from build123d import *

# Parameters (mm, degrees)
AUFSATZ_LINEAR_AUSTRAGEN1_DEPTH  = 20
SCHNITT_LINEAR_AUSTRAGEN2_REACH  = 2.5
SKIZZE8_W                        = 11
SKIZZE8_H                        = 5
AUFSATZ_LINEAR_AUSTRAGEN3_DEPTH  = 8.34
SCHNITT_LINEAR_AUSTRAGEN3_REACH  = 19.821
SKIZZE12_W                       = 1.5
SKIZZE12_H                       = 2
AUFSATZ_LINEAR_AUSTRAGEN4_DEPTH  = 3.98
AUFSATZ_LINEAR_AUSTRAGEN5_DEPTH  = 2.67
AUFSATZ_LINEAR_AUSTRAGEN6_DEPTH  = 2.67
SCHNITT_LINEAR_AUSTRAGEN4_REACH  = 23.901
SKIZZE17_W                       = 3
SKIZZE17_H                       = 16.288675134
AUFSATZ_LINEAR_AUSTRAGEN15_DEPTH = 6.65
SCHNITT_LINEAR_AUSTRAGEN5_REACH  = 14.32


with BuildPart() as part:
    # Skizze1 → Aufsatz-Linear austragen1 (new body)
    with BuildSketch(Plane(origin=(0, 0, 0), x_dir=(1, 0, 0), z_dir=(0, 1, 0))):
        Polygon((5.5, -4.17), (-5.5, -4.17), (-5.5, -1.5), (-7.5, -1.5), (-7.5, 1.5), (-5.5, 1.5), (-5.5, 4.17), (5.5, 4.17), (5.5, 1.5), (7.5, 1.5), (7.5, -1.5), (5.5, -1.5), align=None)
        Polygon((-5, 1), (-5, 3.67), (5, 3.67), (5, 1), (7, 1), (7, -1), (5, -1), (5, -3.67), (-5, -3.67), (-5, -1), (-7, -1), (-7, 1), align=None, mode=Mode.SUBTRACT)
    extrude(amount=AUFSATZ_LINEAR_AUSTRAGEN1_DEPTH)

    # Skizze8 → Schnitt-Linear austragen2 (cut, up to next)
    with BuildSketch(Plane(origin=(0, 0, 3.67), x_dir=(-1, 0, 0), z_dir=(0, 0, -1)), mode=Mode.PRIVATE) as schnitt_linear_austragen2_sk1:
        with Locations((0, 2.5)):
            Rectangle(SKIZZE8_W, SKIZZE8_H)
    schnitt_linear_austragen2_tool1 = extrude(schnitt_linear_austragen2_sk1.sketch, amount=-SCHNITT_LINEAR_AUSTRAGEN2_REACH, mode=Mode.PRIVATE) & part.part
    add(schnitt_linear_austragen2_tool1.solids().sort_by_distance((0, 2.5, 3.67))[0], mode=Mode.SUBTRACT)

    # Skizze10 → Aufsatz-Linear austragen3 (add)
    with BuildSketch(Plane(origin=(0, 0, -4.17), x_dir=(-1, 0, 0), z_dir=(0, 0, -1))):
        Polygon((5.5, 20), (7.211324865, 20), (17.211324865, 37.320508076), (17.644337567, 37.070508076), (7.5, 19.5), (5.5, 19.5), align=None)
    extrude(amount=-AUFSATZ_LINEAR_AUSTRAGEN3_DEPTH)

    # Skizze12 → Schnitt-Linear austragen3 (cut, up to next)
    with BuildSketch(Plane.XZ.offset(-19.5), mode=Mode.PRIVATE) as schnitt_linear_austragen3_sk1:
        with Locations((-6.25, 0)):
            Rectangle(SKIZZE12_W, SKIZZE12_H)
    schnitt_linear_austragen3_tool1 = extrude(schnitt_linear_austragen3_sk1.sketch, amount=-SCHNITT_LINEAR_AUSTRAGEN3_REACH, mode=Mode.PRIVATE) & part.part
    add(schnitt_linear_austragen3_tool1.solids().sort_by_distance((-6.25, 19.5, 0))[0], mode=Mode.SUBTRACT)

    # Skizze13 → Aufsatz-Linear austragen4 (add)
    with BuildSketch(Plane(origin=(0, 0, -4.17), x_dir=(-1, 0, 0), z_dir=(0, 0, -1))):
        Polygon((17.211324865, 37.320508076), (9.561324865, 24.070319398), (9.994337567, 23.820319398), (17.644337567, 37.070508076), align=None)
    aufsatz_linear_austragen4 = extrude(amount=AUFSATZ_LINEAR_AUSTRAGEN4_DEPTH)

    # Skizze15 → Aufsatz-Linear austragen5 (add)
    with BuildSketch(Plane(origin=(0, 0, -1.5), x_dir=(-1, 0, 0), z_dir=(0, 0, -1))):
        Polygon((5.5, 8), (5.5, 19.5), (7.5, 19.5), (17.644337567, 37.070508076), (7.5, 8), align=None)
    extrude(amount=AUFSATZ_LINEAR_AUSTRAGEN5_DEPTH)

    # Spiegeln1: Aufsatz-Linear austragen4 across plane
    add(aufsatz_linear_austragen4.mirror(Plane.XY))

    # Skizze16 → Aufsatz-Linear austragen6 (add)
    with BuildSketch(Plane.XY.offset(1.5)):
        Polygon((-17.644337567, 37.070508076), (-7.5, 8), (-5.5, 8), (-5.5, 19.5), (-7.5, 19.5), align=None)
    extrude(amount=AUFSATZ_LINEAR_AUSTRAGEN6_DEPTH)

    # Skizze17 → Schnitt-Linear austragen4 (cut, up to next)
    with BuildSketch(Plane(origin=(2.818747687, 1.627404736, 0), x_dir=(0, 0, 1), z_dir=(-0.866025404, -0.5, 0)), mode=Mode.PRIVATE) as schnitt_linear_austragen4_sk1:
        with Locations((0, 28.781832941)):
            Rectangle(SKIZZE17_W, SKIZZE17_H)
    schnitt_linear_austragen4_tool1 = extrude(schnitt_linear_austragen4_sk1.sketch, amount=-SCHNITT_LINEAR_AUSTRAGEN4_REACH, mode=Mode.PRIVATE) & part.part
    add(schnitt_linear_austragen4_tool1.solids().sort_by_distance((-11.572169, 26.553203, 0))[0], mode=Mode.SUBTRACT)

    # Skizze22 → Aufsatz-Linear austragen15 (add)
    with BuildSketch(Plane.XY.offset(-1.5)):
        Polygon((-17.611390326, 36.976091556), (-12.603409607, 22.624780496), (-13.075492208, 22.460044288), (-18.083472926, 36.811355348), align=None)
    aufsatz_linear_austragen15 = extrude(amount=-AUFSATZ_LINEAR_AUSTRAGEN15_DEPTH)

    # Spiegeln2: Aufsatz-Linear austragen15 across plane
    add(aufsatz_linear_austragen15.mirror(Plane.XY))

    # Skizze23 → Schnitt-Linear austragen5 (cut, up to next)
    with BuildSketch(Plane.XY.offset(4.17), mode=Mode.PRIVATE) as schnitt_linear_austragen5_sk1:
        Polygon((-7.211324865, 20), (-9.561324865, 20), (-9.561324865, 24.070319398), align=None)
    schnitt_linear_austragen5_tool1 = extrude(schnitt_linear_austragen5_sk1.sketch, amount=-SCHNITT_LINEAR_AUSTRAGEN5_REACH, mode=Mode.PRIVATE) & part.part
    add(schnitt_linear_austragen5_tool1.solids().sort_by_distance((-8.777992, 21.356773, 4.17))[0], mode=Mode.SUBTRACT)


solid = part.part
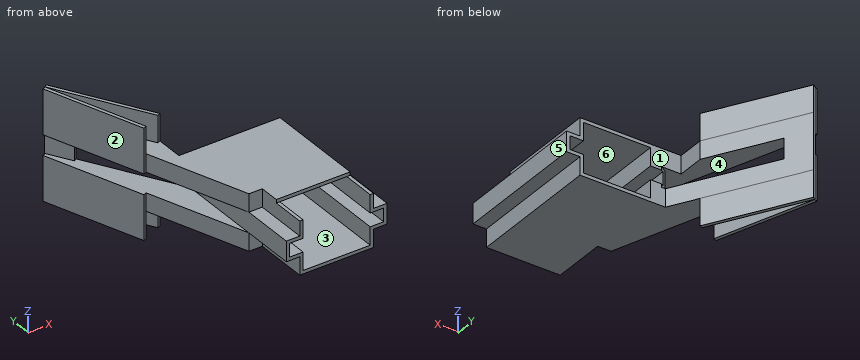
Verification items for the finished model (mm, model axes). Face numbers are marked on the shaded views. A direction names the side the tool comes from. Coordinates: 2 decimals unless noted, no trailing zeros. Order: outer loops, then holes, each group sorted by start corner. A loop starts at its lowest first (then second) coordinate and runs counter-clockwise, first axis right, second up. Notation, with made-up numbers: M 2.25,41 L 50.25,41 A21 cw 50.25,64 Z; hole C 72.5,66 d1. An arc over 180 degrees is marked long. One line per item, written item: value. Start each with the question number.
Item 1: Sectioned sample at B-B (z = -3). Enter the section's corners in (x, y).
Item 2: Sectioned sample at C-C (x = -3). Enter the section's corners in (y, z), then the cut area to 3 significant figures.
Item 3: Gauge pin test, flat ends, axial feed: pin 1 (0.8 mm diameter, centred on y = 10, z = 3, fed in from -X); pin 2 (0.8 mm diameter, centred on y = 22, z = 3, fed in from +X); pin 3 (1 mm diameter, centred on y = 29, z = 0, fed in from +X); pin 4 (8 mm diameter, centred on y = 32, z = -5.5, fed in from -X). Record the tip position at first contact, or that the pin passes through.
Item 4: Scan lines: probe 1 along X at (y, z) = (18, 0.5); probe 2 along X at (y, z) = (3.5, -1.25); probe 3 along Z at (x, y) = (-3.5, 12). Record each from-to range of solid material in increasing order.
Item 5: Mould release check, pull along X, two halves, no side actions. Record for the marked faces 3, 4, 5 and 6: released by +X, released by -X, zero draft, split by the parting line, or undercut.
Item 6: Access from +Z, -Z, +X, -X, +Y, -Y to the whole of each face (thin tool, end or side, straight path). Record for the marked faces 1 and 2.
Item 7: Sectioned sample at A-A (y = 7). Enter the section's corners in (x, z).
Item 8: Sectioned sample at D-D (y = 28.5). Enter the section's corners in (x, z), then the cut area to 3 significant figures.
Conclusion:
1. outline: M -18.08,36.81 L -13.08,22.46 L -12.6,22.62 L -7.5,8 L -5.5,8 L -5.5,0 L -5,0 L -5,20 L -7.21,20 L -17.21,37.32 L -17.64,37.07 L -17.61,36.98 Z; M 5,0 L 5.5,0 L 5.5,20 L 5,20 Z
2. outline: M 0,-4.17 L 20,-4.17 L 20,-3.67 L 0,-3.67 Z; M 5,3.67 L 20,3.67 L 20,4.17 L 5,4.17 Z
2. area: 17.5 mm^2
3. pin 1: stops at x = -8.34
3. pin 2: stops at x = -9.56
3. pin 3: passes through
3. pin 4: stops at x = -17.8
4. probe 1: x = -7.5 to -7, 7 to 7.5
4. probe 2: x = -7.5 to -5, 5 to 7.5
4. probe 3: z = -4.17 to -3.67, 3.67 to 4.17
5. face 3: undercut
5. face 4: zero draft
5. face 5: released by +X
5. face 6: undercut
6. face 1: +Z, +X, +Y
6. face 2: +Z, -Z, -X, -Y
7. outline: M -7.5,-1.5 L -5.5,-1.5 L -5.5,-4.17 L 5.5,-4.17 L 5.5,-1.5 L 7.5,-1.5 L 7.5,1.5 L 5.5,1.5 L 5.5,4.17 L -5.5,4.17 L -5.5,1.5 L -7.5,1.5 Z; hole M -7,-1 L -5,-1 L -5,-3.67 L 5,-3.67 L 5,-1 L 7,-1 L 7,1 L 5,1 L 5,3.67 L -5,3.67 L -5,1 L -7,1 Z
8. outline: M -15.18,-8.15 L -14.65,-8.15 L -14.65,-4.17 L -12.7,-4.17 L -12.7,-8.15 L -12.12,-8.15 L -12.12,-1.5 L -15.18,-1.5 Z; M -15.18,1.5 L -12.12,1.5 L -12.12,8.15 L -12.7,8.15 L -12.7,4.17 L -14.65,4.17 L -14.65,8.15 L -15.18,8.15 Z
8. area: 25.2 mm^2
